```python
from build123d import *

# Parameters (mm, degrees)
CROQUIS1_W                = 12
CROQUIS1_H                = 15
CROQUIS1_W_2              = 8
CROQUIS1_H_2              = 11
SALIENTE_EXTRUIR1_DEPTH   = 176.5
CROQUIS3_R                = 2.5
SALIENTE_EXTRUIR2_DEPTH   = 2
SIMETR_A2_COPY_1_SKETCH_R = 2.5
SIMETR_A2_COPY_1_DEPTH    = 2
SKETCH1_R                 = 2.5
CUT_EXTRUDE1_DEPTH        = 28
SKETCH6_W                 = 176.5
SKETCH6_H                 = 30.622513857
CUT_EXTRUDE2_DEPTH        = 15
SKETCH7_W                 = 10
SKETCH7_H                 = 20.073339824
CUT_EXTRUDE3_DEPTH        = 10
SKETCH8_R                 = 2.5
CUT_EXTRUDE4_DEPTH        = 15


with BuildPart() as part:
    # Croquis1 → Saliente-Extruir1 (new body, symmetric)
    with BuildSketch(Plane.XY):
        Rectangle(CROQUIS1_W, CROQUIS1_H)
        Rectangle(CROQUIS1_W_2, CROQUIS1_H_2, mode=Mode.SUBTRACT)
    extrude(amount=SALIENTE_EXTRUIR1_DEPTH, both=True)

    # Croquis3 → Saliente-Extruir2 (add)
    with BuildSketch(Plane.ZY.offset(6)):
        with BuildLine():
            Line((-145, -14.5), (-145, -0.5))
            Line((-145, -0.5), (-135, -0.5))
            Line((-135, -0.5), (-135, -14.5))
            ThreePointArc((-135, -14.5), (-140, -19.5), (-145, -14.5))
        make_face()
        with Locations((-140, -14.5)):
            Circle(CROQUIS3_R, mode=Mode.SUBTRACT)
    saliente_extruir2 = extrude(amount=SALIENTE_EXTRUIR2_DEPTH)

    # Simetría1: Saliente-Extruir2 across plane
    add(saliente_extruir2.mirror(Plane(origin=(0, 0, 0), x_dir=(0, 0, 1), z_dir=(1, 0, 0))))

    # Simetría2: Saliente-Extruir2 across plane
    add(saliente_extruir2.mirror(Plane.XY))

    # Simetría2 copy 1 sketch → Simetría2 copy 1 (add)
    with BuildSketch(Plane(origin=(6, 0, 0), x_dir=(0, 0, -1), z_dir=(1, 0, 0))):
        with BuildLine():
            Line((-145, -14.5), (-145, -0.5))
            Line((-145, -0.5), (-135, -0.5))
            Line((-135, -0.5), (-135, -14.5))
            ThreePointArc((-135, -14.5), (-140, -19.5), (-145, -14.5))
        make_face()
        with Locations((-140, -14.5)):
            Circle(SIMETR_A2_COPY_1_SKETCH_R, mode=Mode.SUBTRACT)
    extrude(amount=SIMETR_A2_COPY_1_DEPTH)

    # Sketch1 → Cut-Extrude1 (cut, through all)
    with BuildSketch(Plane(origin=(0, 7.5, 0), x_dir=(1, 0, 0), z_dir=(0, 1, 0))):
        with Locations((0, 170.5)):
            Circle(SKETCH1_R)
        with Locations((0, -170.5)):
            Circle(SKETCH1_R)
    extrude(amount=-CUT_EXTRUDE1_DEPTH, mode=Mode.SUBTRACT)

    # Sketch6 → Cut-Extrude2 (cut, through all)
    with BuildSketch(Plane.ZY.offset(6)):
        with Locations((-88.25, -7.811256929)):
            Rectangle(SKETCH6_W, SKETCH6_H)
    extrude(amount=-CUT_EXTRUDE2_DEPTH, mode=Mode.SUBTRACT)

    # Sketch7 → Cut-Extrude3 (cut)
    with BuildSketch(Plane.ZY.offset(8)):
        with Locations((-140, -10.536669912)):
            Rectangle(SKETCH7_W, SKETCH7_H)
    extrude(amount=-CUT_EXTRUDE3_DEPTH, mode=Mode.SUBTRACT)

    # Sketch8 → Cut-Extrude4 (cut, through all)
    with BuildSketch(Plane(origin=(6, 0, 0), x_dir=(0, 0, -1), z_dir=(1, 0, 0))):
        with Locations((-9, 1)):
            Circle(SKETCH8_R)
    extrude(amount=-CUT_EXTRUDE4_DEPTH, mode=Mode.SUBTRACT)


solid = part.part
```
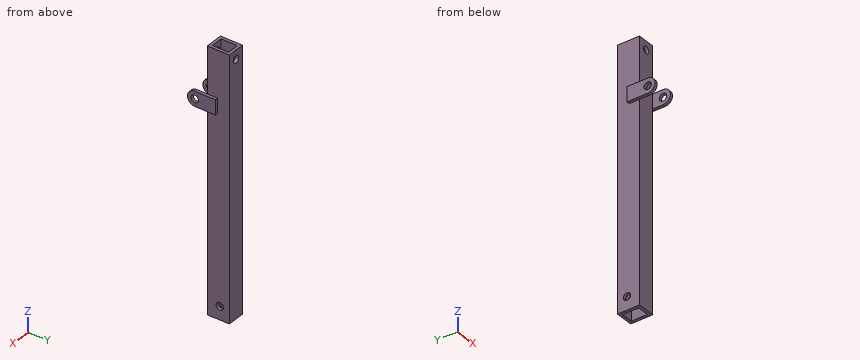
Design review of the part built by this model. Coordinates are the model's own, in mm. Coordinates: 2 decimals unless noted, no trailing zeros. Write each loop counter-clockwise with the first axis right and the second up, starting at its lowest first coordinate (ties: lowest second). Pieces come first, ordered by that corner, then holes.
1) Insertion check: pin 1 (6 mm diameter, centred on x = 0, z = 170.5, fed in from -Y); pin 2 (4 mm diameter, centred on x = 4.5, y = -15.5, fed in from +Z); pin 3 (1.6 mm diameter, centred on x = -6.5, y = -5, fed in from +Z); pin 4 (5.5 mm diameter, centred on y = 1, z = 77.5, fed in from -X). Each pin has a flat end and moves straight along its axis. Give the tip position at first contact, or say it passes through.
2) To check wall thickness, follow L1, parallel to Z at x = 0, y = -6.1; L2, parallel to Y at x = -3.25, z = 159.5; L3, parallel to Y at x = 7.4, z = 140. State the ranges of each line that lie inside material, in increasing order.
3) Add section C-C (x = 0). Write out the cut boundary in (y, z), plus the area to 3 significant figures.
4) Add section D-D (z = 9). Write out the cut boundary in (x, y), plus the area to 3 significant figures.
5) Add section B-B (y = 1). Write out the cut boundary in (x, z).
6) Add section A-A (z = 140). Write out the cut boundary in (x, y).
Check result:
1. pin 1: stops at y = -7.5
1. pin 2: stops at z = 145
1. pin 3: stops at z = 176.5
1. pin 4: stops at x = -6
2. L1: z = 0 to 168, 173 to 176.5
2. L2: y = -7.5 to -5.5, 5.5 to 7.5
2. L3: y = -19.5 to -17, -12 to -0.5
3. outline: (-7.5, 0) - (-5.5, 0) - (-5.5, 168) - (-7.5, 168) - close; (-7.5, 173) - (-5.5, 173) - (-5.5, 176.5) - (-7.5, 176.5) - close; (5.5, 0) - (7.5, 0) - (7.5, 168) - (5.5, 168) - close; (5.5, 173) - (7.5, 173) - (7.5, 176.5) - (5.5, 176.5) - close
3. area: 686 mm2
4. outline: (-6, -7.5) - (6, -7.5) - (6, -1.5) - (4, -1.5) - (4, -5.5) - (-4, -5.5) - (-4, -1.5) - (-6, -1.5) - close; (-6, 3.5) - (-4, 3.5) - (-4, 5.5) - (4, 5.5) - (4, 3.5) - (6, 3.5) - (6, 7.5) - (-6, 7.5) - close
4. area: 72.0 mm2
5. outline: (-6, 0) - (-4, 0) - (-4, 6.5) - (-6, 6.5) - close; (-6, 11.5) - (-4, 11.5) - (-4, 176.5) - (-6, 176.5) - close; (4, 0) - (6, 0) - (6, 6.5) - (4, 6.5) - close; (4, 11.5) - (6, 11.5) - (6, 176.5) - (4, 176.5) - close
6. outline: (-8, -19.5) - (-6, -19.5) - (-6, -17) - (-8, -17) - close; (-8, -12) - (-6, -12) - (-6, -7.5) - (6, -7.5) - (6, -12) - (8, -12) - (8, -0.5) - (6, -0.5) - (6, 7.5) - (-6, 7.5) - (-6, -0.5) - (-8, -0.5) - close; (6, -19.5) - (8, -19.5) - (8, -17) - (6, -17) - close; hole (-4, -5.5) - (4, -5.5) - (4, 5.5) - (-4, 5.5) - close
